Build history of the part. All positions in model axes, mm. A direction names the side the tool comes from. Round coordinates to 2 decimals unless told otherwise and drop trailing zeros. Loops run counter-clockwise (first coordinate to the right, second up) from the corner with the lowest first, then second, coordinate; pieces in that order, holes last. Notation, with made-up numbers: (-22, 83.25) - (-15, 83.25) arc R32 ccw to (-15, 117.25) - close; hole circle Ø5 at (-33, -24.75). An arc over 180 degrees is marked (long way). Put each result on its own line as item: value. Start each with the question number.
from build123d import *

# Parameters (mm, degrees)
TAGLIO_ESTRUSIONE1_REACH                  = 43.569
TAGLIO_ESTRUSIONE1_END_RADIUS             = 8
SCHIZZO2_W                                = 1.5
SCHIZZO2_H                                = 8
TAGLIO_ESTRUSIONE1_DIRECTION_2_REACH      = 43.569
TAGLIO_ESTRUSIONE1_DIRECTION_2_END_RADIUS = 8
SCHIZZO7_R                                = 3
TAGLIO_ESTRUSIONE2_DEPTH                  = 42.569219382
FORO_FILETTATO_M8_1_D                     = 6.8
FORO_FILETTATO_M8_1_DEPTH                 = 12
FORO_FILETTATO_M8_1_TIP                   = 2.042926105
TAGLIO_ESTRUSIONE3_REACH                  = 43.569
SCHIZZO10_R                               = 8
SCHIZZO10_R_2                             = 7
ESTRUSIONE_ESTRUSIONE1_START              = 4.6
SCHIZZO11_R                               = 7
ESTRUSIONE_ESTRUSIONE1_DEPTH              = 4.6
SCHIZZO12_R                               = 3
TAGLIO_ESTRUSIONE4_DEPTH                  = 5


with BuildPart() as part:
    # Schizzo1 → Rivoluzione1 (revolve)
    with BuildSketch(Plane.XY, mode=Mode.PRIVATE) as rivoluzione1_sk:
        Polygon((0, 0), (-5, 0), (-8, 1.5), (-8, 12), (-6, 12), (-6, 13.5), (-8, 13.5), (-8, 15), (-6, 15), (-6, 16.5), (-8, 16.5), (-8, 18), (-6, 18), (-6, 19.5), (-8, 19.5), (-8, 30.6), (-6, 30.6), (-6, 35.2), (-8, 35.2), (-8, 40), (0, 40), align=None)
    revolve(rivoluzione1_sk.sketch.rotate(Axis((0, 129.407380346, 0), (0, -1, 0)), 270), axis=Axis((0, 129.407380346, 0), (0, -1, 0)))

    # Taglio-Estrusione1: up to this cylinder (the profile starts inside it)
    taglio_estrusione1_end = Plane(origin=(0, 4, 0), z_dir=(0, 1, 0)) * Cylinder(TAGLIO_ESTRUSIONE1_END_RADIUS, 104.138, mode=Mode.PRIVATE)
    # Schizzo2 → Taglio-Estrusione1 (cut, up to the surface)
    with BuildSketch(Plane.XY, mode=Mode.PRIVATE) as taglio_estrusione1_sk1:
        with Locations((-7.25, 4)):
            Rectangle(SCHIZZO2_W, SCHIZZO2_H)
    taglio_estrusione1_tool1 = extrude(taglio_estrusione1_sk1.sketch, amount=-TAGLIO_ESTRUSIONE1_REACH, mode=Mode.PRIVATE) & taglio_estrusione1_end
    add(taglio_estrusione1_tool1.solids().sort_by_distance((-7.25, 4, 0))[0], mode=Mode.SUBTRACT)
    # Schizzo2 → Taglio-Estrusione1 (cut, up to the surface)
    with BuildSketch(Plane.XY, mode=Mode.PRIVATE) as taglio_estrusione1_sk2:
        with Locations((7.25, 4)):
            Rectangle(SCHIZZO2_W, SCHIZZO2_H)
    taglio_estrusione1_tool2 = extrude(taglio_estrusione1_sk2.sketch, amount=-TAGLIO_ESTRUSIONE1_REACH, mode=Mode.PRIVATE) & taglio_estrusione1_end
    add(taglio_estrusione1_tool2.solids().sort_by_distance((7.25, 4, 0))[0], mode=Mode.SUBTRACT)

    # Taglio-Estrusione1 direction 2: up to this cylinder (the profile starts inside it)
    taglio_estrusione1_direction_2_end = Plane(origin=(0, 4, 0), z_dir=(0, 1, 0)) * Cylinder(TAGLIO_ESTRUSIONE1_DIRECTION_2_END_RADIUS, 104.138, mode=Mode.PRIVATE)
    # Schizzo2 → Taglio-Estrusione1 direction 2 (cut, up to the surface)
    with BuildSketch(Plane.XY, mode=Mode.PRIVATE) as taglio_estrusione1_direction_2_sk1:
        with Locations((-7.25, 4)):
            Rectangle(SCHIZZO2_W, SCHIZZO2_H)
    taglio_estrusione1_direction_2_tool1 = extrude(taglio_estrusione1_direction_2_sk1.sketch, amount=TAGLIO_ESTRUSIONE1_DIRECTION_2_REACH, mode=Mode.PRIVATE) & taglio_estrusione1_direction_2_end
    add(taglio_estrusione1_direction_2_tool1.solids().sort_by_distance((-7.25, 4, 0))[0], mode=Mode.SUBTRACT)
    # Schizzo2 → Taglio-Estrusione1 direction 2 (cut, up to the surface)
    with BuildSketch(Plane.XY, mode=Mode.PRIVATE) as taglio_estrusione1_direction_2_sk2:
        with Locations((7.25, 4)):
            Rectangle(SCHIZZO2_W, SCHIZZO2_H)
    taglio_estrusione1_direction_2_tool2 = extrude(taglio_estrusione1_direction_2_sk2.sketch, amount=TAGLIO_ESTRUSIONE1_DIRECTION_2_REACH, mode=Mode.PRIVATE) & taglio_estrusione1_direction_2_end
    add(taglio_estrusione1_direction_2_tool2.solids().sort_by_distance((7.25, 4, 0))[0], mode=Mode.SUBTRACT)

    # Schizzo7 → Taglio-Estrusione2 (cut, through all)
    with BuildSketch(Plane(origin=(0, 40, 0), x_dir=(1, 0, 0), z_dir=(0, 1, 0))):
        with Locations(Location((0, 0, 0), (0, 0, 270))):
            Circle(SCHIZZO7_R)
    extrude(amount=-TAGLIO_ESTRUSIONE2_DEPTH, mode=Mode.SUBTRACT)

    # Foro filettato M8-1
    with Locations(Plane(origin=(0, 0, 0), x_dir=(-1, 0, 0), z_dir=(0, -1, 0))):
        with Locations((0, 0)):
            Hole(FORO_FILETTATO_M8_1_D / 2, depth=FORO_FILETTATO_M8_1_DEPTH)
            with Locations((0, 0, -(FORO_FILETTATO_M8_1_DEPTH + FORO_FILETTATO_M8_1_TIP / 2))):  # 118° drill point
                Cone(0, FORO_FILETTATO_M8_1_D / 2, FORO_FILETTATO_M8_1_TIP, mode=Mode.SUBTRACT)

    # Taglio-Estrusione3: up to this face of the body (flat: up to its plane)
    taglio_estrusione3_end = Plane(part.part.faces().sort_by_distance((0, 0, -4.858578644))[0])
    # Schizzo10 → Taglio-Estrusione3 (cut, up to the picked face)
    with BuildSketch(Plane(origin=(0, 40, 0), x_dir=(1, 0, 0), z_dir=(0, 1, 0)), mode=Mode.PRIVATE) as taglio_estrusione3_sk1:
        Circle(SCHIZZO10_R)
        with Locations(Location((0, 0, 0), (0, 0, 270))):
            Circle(SCHIZZO10_R_2, mode=Mode.SUBTRACT)
    taglio_estrusione3_tool1 = split(extrude(taglio_estrusione3_sk1.sketch, amount=-TAGLIO_ESTRUSIONE3_REACH, mode=Mode.PRIVATE), bisect_by=taglio_estrusione3_end, keep=Keep.BOTH, mode=Mode.PRIVATE)
    add(taglio_estrusione3_tool1.solids().sort_by(Axis((-7.773726, 40, 0), (0, -1, 0)))[0], mode=Mode.SUBTRACT)

    # Schizzo11 → Estrusione-Estrusione1 (add)
    with BuildSketch(Plane(origin=(0, 30.6, 0), x_dir=(1, 0, 0), z_dir=(0, 1, 0)).offset(ESTRUSIONE_ESTRUSIONE1_START)):
        with Locations(Location((0, 0, 0), (0, 0, 270))):
            Circle(SCHIZZO11_R)
    extrude(amount=-ESTRUSIONE_ESTRUSIONE1_DEPTH)

    # Schizzo12 → Taglio-Estrusione4 (cut)
    with BuildSketch(Plane(origin=(0, 35.2, 0), x_dir=(1, 0, 0), z_dir=(0, 1, 0))):
        with Locations(Location((0, 0, 0), (0, 0, 270))):
            Circle(SCHIZZO12_R)
    extrude(amount=-TAGLIO_ESTRUSIONE4_DEPTH, mode=Mode.SUBTRACT)


solid = part.part
Item 1: Drop flat-ended pins along their axis: pin 1 Ø1.5 at (x, y) = (3.5, 11.5) entering from -Z; pin 2 Ø5.5 at (y, z) = (4, 0) entering from +X; pin 3 Ø7 at (x, z) = (2.5, -3) entering from -Y; pin 4 Ø0.6 at (x, z) = (6.5, 0.5) entering from -Y. Give the stop position or say it passes through.
Item 2: Slice it at B-B (y = 37). Give the cut face in (x, z).
Item 3: Slice it at A-A (y = 6.5). Give the cut face in (x, z), plus the area to 3 significant figures.
Item 4: Drill centre lines: probe 1 along Z at (x, y) = (-0.25, 7); probe 2 along X at (y, z) = (31.5, 0); probe 3 along Y at (x, z) = (3, 5.5). Where is each one in solid material? Low to high. Write a range as [from, to].
Item 5: Which spindle directions (+Z, -Z, +X, -X, +Y, -Y) get a long thin tool onto all of the face, cutting with end or side? Do faces 1 (the cylindrical face through (-2.681, 6.577, 6.466)), 2 (the flat face through (6.5, 4, 0)), 3 (the flat face through (-2, 12, 6)). Say none if no direction does.
Item 6: Two-plate mould, pull along X, no slides. Class faces 4 (the cylindrical face through (0.9, 26.31, 2.86)), 5 (the flat face through (-2, 18, 6)), 6 (the flat face through (-6.5, 4, 0)), 7 (the cylindrical face through (-0.74, 6.08, 3.32)): pulls with the +X half, pulls with the -X half, needs draft (parallel to the pull), parting line crosses it, or undercut.
Computed values:
1. pin 1: stops at z = -6.44
1. pin 2: stops at x = 6.5
1. pin 3: stops at y = 0
1. pin 4: stops at y = 0.61
2. outline: circle Ø14 at (0, 0); hole circle Ø6 at (0, 0)
3. outline: (-6.5, -2.6) arc R7 ccw to (6.5, -2.6) - (6.5, 2.6) arc R7 ccw to (-6.5, 2.6) - close; hole circle Ø6.8 at (0, 0)
3. area: 114 mm^2
4. probe 1: z = [-7, -3.39], [3.39, 7]
4. probe 2: x = [-7, -3], [3, 7]
4. probe 3: y = [0.63, 12], [13.5, 15], [16.5, 18], [19.5, 40]
5. face 1: +Y, -Y
5. face 2: +Z, -Z, +X, -Y
5. face 3: none
6. face 4: undercut
6. face 5: needs draft
6. face 6: pulls with the -X half
6. face 7: undercut
